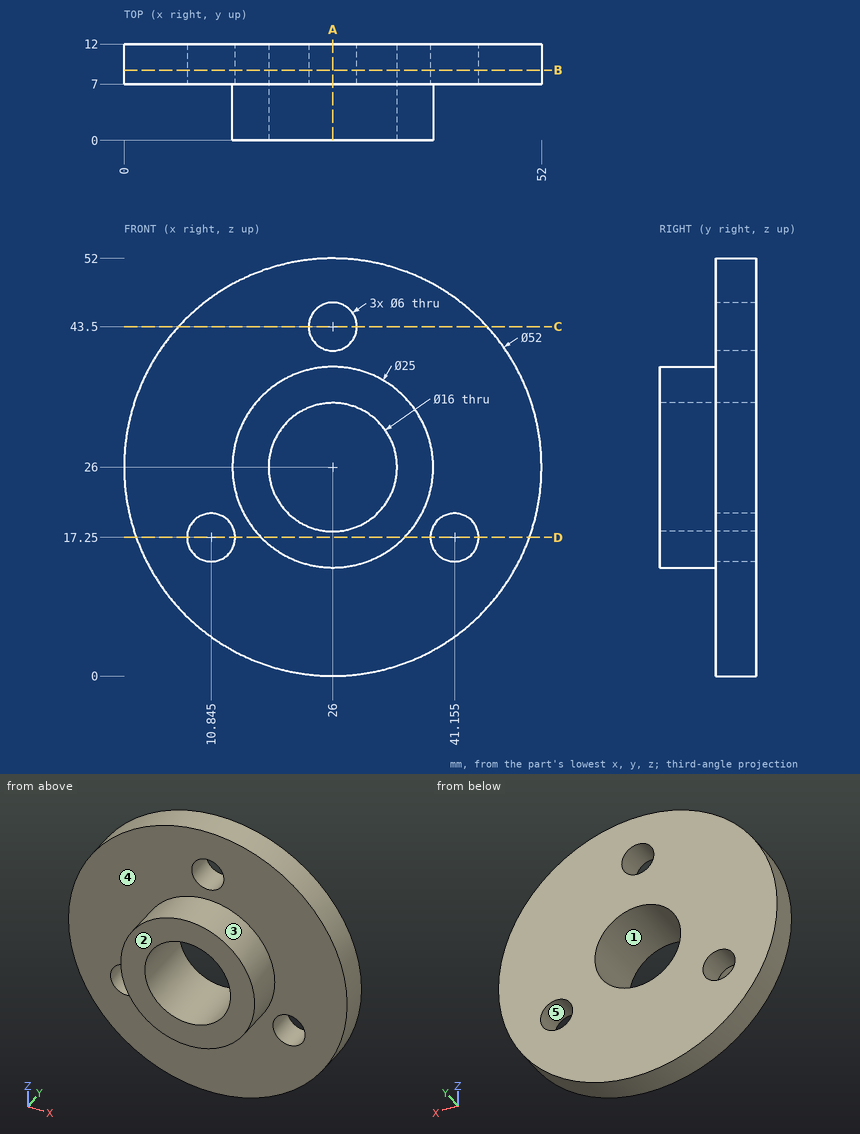
Answer from the drawing. Dimensions are ordinates in mm from the lowest x, y and z of the part. A direction names the side the tool comes from. Give positions to 0.01 mm unless a question says otherwise; leave off trailing zeros. Loops run counter-clockwise (first coordinate to the right, second up) from the corner with the lowest first, then second, coordinate; pieces in that order, holes last.
Item 1: A tool of negligible diameter and unlimited length cuts with its end or side. For the marked faces 4 and 5, from which of +Z, -Z, +X, -X, +Y, -Y can it reach the whole face along a straight path? Write none if from no direction.
Derived:
face 4: -Y
face 5: +Y, -Y
Item 2: Each of these flat-tipped pins is pushed along its axis until it touches: pin 1 Ø2 at (x, y) = (38, 4) entering from -Z (1 decimal); pin 2 Ø7 at (x, z) = (41.16, 17.25) entering from -Y; pin 3 Ø3 at (y, z) = (3.5, 19.5) entering from -X. Where does it stop, or does it pass through?
Derived:
pin 1: stops at z = 20.1
pin 2: stops at y = 7
pin 3: stops at x = 14.54
Item 3: Find the intervals of material crossed by line 1 along Z through (x, y) = (24, 11) (1 decimal); line 2 along Z through (x, y) = (25.5, 9) (1 decimal); line 3 along Y through (x, z) = (8.5, 27.5), in increasing order.
Derived:
line 1: z = 0.1 to 18.3, 33.7 to 41.3, 45.7 to 51.9
line 2: z = 0 to 18, 34 to 40.5, 46.5 to 52
line 3: y = 7 to 12
Item 4: A cutting plane is placed at D-D (z = 17.25). Give the vertices of the cut face in (x, y) (1 decimal).
Derived:
outline: (1.5, 7) - (7.8, 7) - (7.8, 12) - (1.5, 12) - close; (13.8, 7) - (17.1, 7) - (17.1, 0) - (34.9, 0) - (34.9, 7) - (38.2, 7) - (38.2, 12) - (13.8, 12) - close; (44.2, 7) - (50.5, 7) - (50.5, 12) - (44.2, 12) - close
Item 5: A cutting plane is placed at B-B (y = 8.75). Give the number of separate pieces and of enclosed holes in the cut face, then the cut area to 3 significant figures.
Derived:
separate pieces: 1
enclosed holes: 4
area: 1,840 mm2
Item 6: A cutting plane is placed at A-A (x = 26). Give the vertices of the cut face in (y, z).
Derived:
outline: (0, 13.5) - (7, 13.5) - (7, 0) - (12, 0) - (12, 18) - (0, 18) - close; (0, 34) - (12, 34) - (12, 40.5) - (7, 40.5) - (7, 38.5) - (0, 38.5) - close; (7, 46.5) - (12, 46.5) - (12, 52) - (7, 52) - close
Item 7: A cutting plane is placed at C-C (z = 43.5). Give the vertices of the cut face in (x, y).
Derived:
outline: (6.77, 7) - (23, 7) - (23, 12) - (6.77, 12) - close; (29, 7) - (45.23, 7) - (45.23, 12) - (29, 12) - close
Item 8: Determine the mould class of the marked faces 1, 2 and 3 for opening direction X: +X half, -X half, draft (parallel to the pull), parting line (faces both ways), or undercut.
Derived:
face 1: undercut
face 2: draft
face 3: parting line
